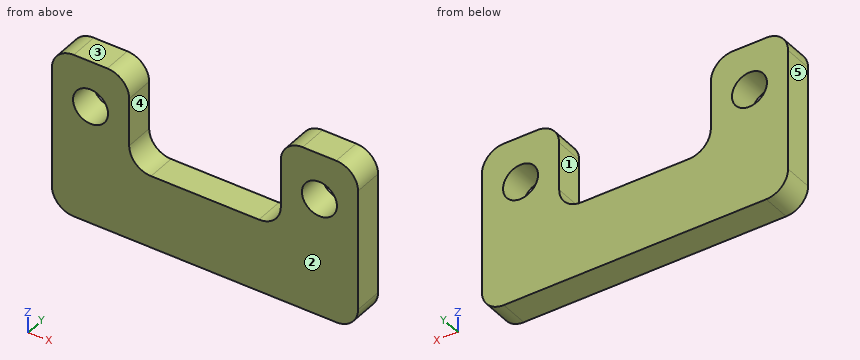
```python
from build123d import *

# Parameters (mm, degrees)
BOSS_EXTRUDE1_DEPTH  = 2
M2_CLEARANCE_HOLE1_D = 2.4
FILLET1_R            = 1.5


with BuildPart() as part:
    # Sketch1 → Boss-Extrude1 (new body)
    with BuildSketch(Plane(origin=(0, 0, 0), x_dir=(1, 0, 0), z_dir=(0, 1, 0))):
        Polygon((-10.5, 2.5), (10.5, 2.5), (10.5, -2.5), (10.5, -8.8), (5.2, -8.8), (5.2, -2.5), (-5.2, -2.5), (-5.2, -8.8), (-10.5, -8.8), (-10.5, -2.5), align=None)
    extrude(amount=BOSS_EXTRUDE1_DEPTH)

    # M2 Clearance Hole1 (through all)
    with Locations(Plane(origin=(0, 2, 0), x_dir=(1, 0, 0), z_dir=(0, 1, 0))):
        with Locations((-7.85, -5.65), (7.85, -5.65)):
            Hole(M2_CLEARANCE_HOLE1_D / 2)

    # Fillet1
    fillet1_edges = [part.edges().sort_by_distance(p)[0] for p in [
        (10.5, 1, 8.8),
        (5.2, 1, 8.8),
        (5.2, 1, 2.5),
        (-5.2, 1, 2.5),
        (-5.2, 1, 8.8),
        (-10.5, 1, 8.8),
        (-10.5, 1, -2.5),
        (10.5, 1, -2.5),
    ]]
    fillet(fillet1_edges, radius=FILLET1_R)


solid = part.part
```
Here's how the part is built. I have some questions about the finished solid (model axes, mm). Face numbers are marked on the shaded views. A direction names the side the tool comes from. Coordinates: 2 decimals unless noted, no trailing zeros. Loops run counter-clockwise (first coordinate to the right, second up) from the corner with the lowest first, then second, coordinate; pieces in that order, holes last. Notation, with made-up numbers: (1.25, 75) -> (47.25, 75) arc R15 cw to (47.25, 85) -> close; hole circle Ø5 at (13.5, 34.25). An arc over 180 degrees is marked (long way). Return JSON: item names as keys, results as strings.
1) If we section it at D-D, the plane z = 3.5: Write out the boundary of the cut face in (x, y).
Results below:
{"outline": "(-10.5, 0) -> (-5.11, 0) -> (-5.11, 2) -> (-10.5, 2) -> close; (5.11, 0) -> (10.5, 0) -> (10.5, 2) -> (5.11, 2) -> close"}
2) Will this pin go through, and if not, where does the flat tip stop? pin 1 (1 mm diameter, centred on x = -1.5, y = 1.5, fed in from +Z).
Results below:
{"pin 1": "z = 2.5"}
3) If we section it at B-B, the plane x = -7.85: Write out the boundary of the cut face in (y, z).
Results below:
{"outline": "(0, -2.5) -> (2, -2.5) -> (2, 4.45) -> (0, 4.45) -> close; (0, 6.85) -> (2, 6.85) -> (2, 8.8) -> (0, 8.8) -> close"}
4) If we section it at A-A, the plane z = 5.65: Write out the boundary of the cut face in (x, y).
Results below:
{"outline": "(-10.5, 0) -> (-9.05, 0) -> (-9.05, 2) -> (-10.5, 2) -> close; (-6.65, 0) -> (-5.2, 0) -> (-5.2, 2) -> (-6.65, 2) -> close; (5.2, 0) -> (6.65, 0) -> (6.65, 2) -> (5.2, 2) -> close; (9.05, 0) -> (10.5, 0) -> (10.5, 2) -> (9.05, 2) -> close"}
5) If we section it at C-C, the plane y = 1.05: Write out the boundary of the cut face in (x, z), then the cut area to 3 significant figures.
Results below:
{"outline": "(-10.5, -1) arc R1.5 ccw to (-9, -2.5) -> (9, -2.5) arc R1.5 ccw to (10.5, -1) -> (10.5, 7.3) arc R1.5 ccw to (9, 8.8) -> (6.7, 8.8) arc R1.5 ccw to (5.2, 7.3) -> (5.2, 4) arc R1.5 cw to (3.7, 2.5) -> (-3.7, 2.5) arc R1.5 cw to (-5.2, 4) -> (-5.2, 7.3) arc R1.5 ccw to (-6.7, 8.8) -> (-9, 8.8) arc R1.5 ccw to (-10.5, 7.3) -> close; hole circle Ø2.4 at (-7.85, 5.65); hole circle Ø2.4 at (7.85, 5.65)", "area": "161 mm²"}
6) For the marked faces 1 and 2, which set-ups out of +Z, -Z, +X, -X, +Y, -Y let a thin tool reach every point of the face, with its end or its side?
Results below:
{"face 1": "+Z, +Y, -Y", "face 2": "+Z, -Z, +X, -X, -Y"}
7) I need wall thicknesses on line 1 (X direction, y = 0.7, z = 5.65); line 2 (Z direction, x = -7.85, y = 0.8); line 3 (X direction, y = 0.7, z = 4). Which ranges of each line are inside material? Lowest first, please. Write a range as from..to.
Results below:
{"line 1": "-10.5..-9.05, -6.65..-5.2, 5.2..6.65, 9.05..10.5", "line 2": "-2.5..4.45, 6.85..8.8", "line 3": "-10.5..-5.2, 5.2..10.5"}
8) Thinking about a two-plate mould opening in X: for the marked faces 3, 4 and 5, which applies, +X half, -X half, draft (parallel to the pull), parting line (faces both ways), or undercut?
Results below:
{"face 3": "draft", "face 4": "undercut", "face 5": "-X half"}
